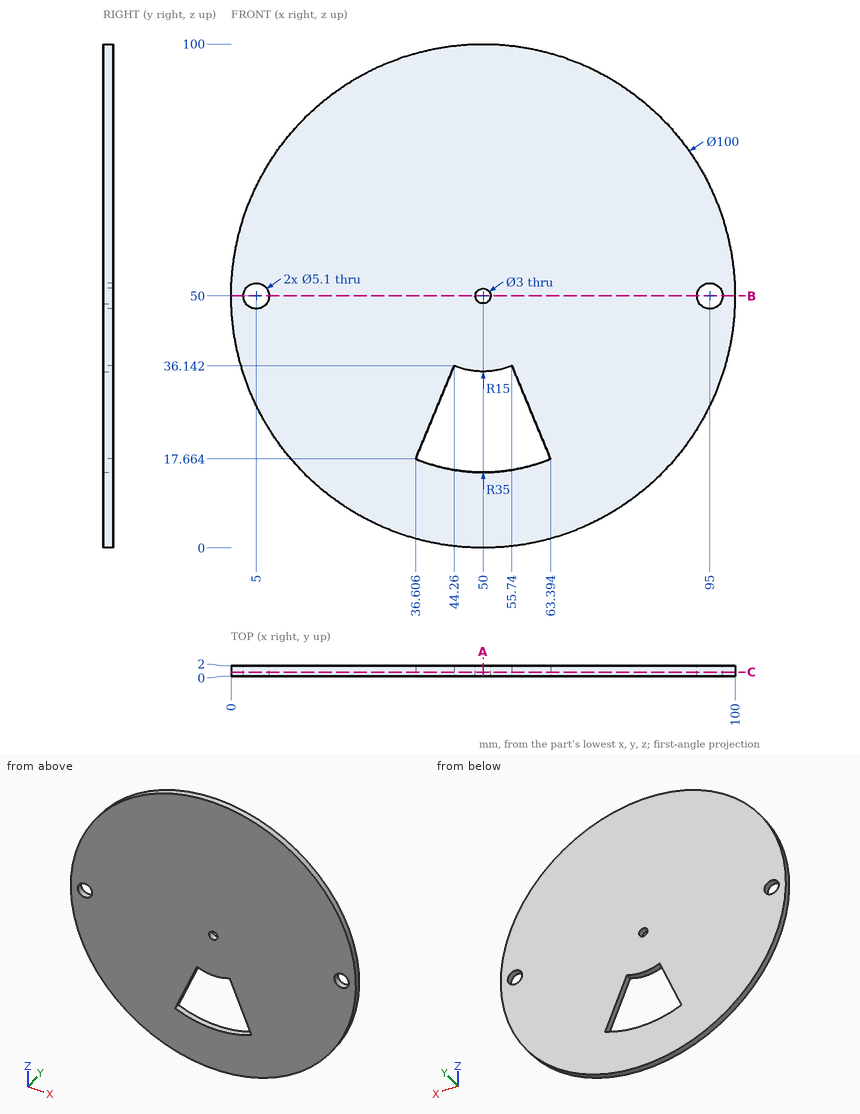
Study the drawing (mm; zero at the part's minimum x, y, z) and answer. Coordinates: 2 decimals unless noted, no trailing zeros. Write each loop counter-clockwise with the first axis right and the second up, starting at its lowest first coordinate (ties: lowest second). Pieces come first, ordered by that corner, then holes. Notation, with made-up numbers: (72.25, 75.25) -> (102.25, 75.25) arc R27 cw to (102.25, 104.25) -> close; hole circle Ø6 at (-32, 89). An arc over 180 degrees is marked (long way). Write item = value, one per line.
(1) Section B-B on z = 50 is taken. Write down the section's boundary in (x, y), plus the area to 3 significant figures.
From the geometry:
outline = (0, 0) -> (2.45, 0) -> (2.45, 2) -> (0, 2) -> close; (7.55, 0) -> (48.5, 0) -> (48.5, 2) -> (7.55, 2) -> close; (51.5, 0) -> (92.45, 0) -> (92.45, 2) -> (51.5, 2) -> close; (97.55, 0) -> (100, 0) -> (100, 2) -> (97.55, 2) -> close
area = 174 mm2
(2) Straight lines are drawn through the part: L1, parallel to X at y = 1.05, z = 50; L2, parallel to Z at x = 51, y = 0.5 (1 decimal); L3, parallel to X at y = 1.65, z = 32 (1 decimal). For each, find the intervals that lie inside material, in ascending order. Write a range as from..to.
From the geometry:
L1 = 0..2.45, 7.55..48.5, 51.5..92.45, 97.55..100
L2 = 0..15, 35..48.9, 51.1..100
L3 = 3.4..42.5, 57.5..96.6
(3) Section A-A on x = 50 is taken. Write down the section's boundary in (y, z), plus the area to 3 significant figures.
From the geometry:
outline = (0, 0) -> (2, 0) -> (2, 15) -> (0, 15) -> close; (0, 35) -> (2, 35) -> (2, 48.5) -> (0, 48.5) -> close; (0, 51.5) -> (2, 51.5) -> (2, 100) -> (0, 100) -> close
area = 154 mm2
(4) Section C-C on y = 0.75 is taken. Write down the section's boundary in (x, z), plus the area to 3 significant figures.
From the geometry:
outline = circle Ø100 at (50, 50); hole circle Ø5.1 at (5, 50); hole (36.61, 17.66) arc R35 ccw to (63.39, 17.66) -> (55.74, 36.14) arc R15 cw to (44.26, 36.14) -> close; hole circle Ø3 at (50, 50); hole circle Ø5.1 at (95, 50)
area = 7,410 mm2
